from build123d import *

# Parameters (mm, degrees)
SKETCH2_R           = 50.8
SKETCH2_R_2         = 49.53
BOSS_EXTRUDE1_DEPTH = 304.8
CUT_EXTRUDE1_REACH  = 67.111
SKETCH3_W           = 80
SKETCH3_H           = 200
SKETCH7_R           = 1.5
CUT_EXTRUDE2_DEPTH  = 10


with BuildPart() as part:
    # Sketch2 → Boss-Extrude1 (new body)
    with BuildSketch(Plane.XY):
        Circle(SKETCH2_R)
        Circle(SKETCH2_R_2, mode=Mode.SUBTRACT)
    extrude(amount=BOSS_EXTRUDE1_DEPTH)

    # Sketch3 → Cut-Extrude1 (cut, up to next)
    with BuildSketch(Plane(origin=(0, 0, 0), x_dir=(0.939692621, -0.342020143, 0), z_dir=(0.342020143, 0.939692621, 0)), mode=Mode.PRIVATE) as cut_extrude1_sk1:
        with Locations((0, -152.4)):
            Rectangle(SKETCH3_W, SKETCH3_H)
    cut_extrude1_tool1 = extrude(cut_extrude1_sk1.sketch, amount=CUT_EXTRUDE1_REACH, mode=Mode.PRIVATE) & part.part
    add(cut_extrude1_tool1.solids().sort_by_distance((0, 0, 152.4))[0], mode=Mode.SUBTRACT)

    # Sketch7 → Cut-Extrude2 (cut)
    with BuildSketch(Plane(origin=(-78.038389788, 6.264218534, 0), x_dir=(-0.785593968, -0.618742367, 0), z_dir=(0.618742367, -0.785593968, 0))):
        with Locations((-57.430550893, -222.4)):
            Circle(SKETCH7_R)
        with Locations((-57.430550893, -197)):
            Circle(SKETCH7_R)
        with Locations((-57.430550893, -107.8)):
            Circle(SKETCH7_R)
        with Locations((-57.430550893, -82.4)):
            Circle(SKETCH7_R)
    extrude(amount=CUT_EXTRUDE2_DEPTH, mode=Mode.SUBTRACT)


solid = part.part
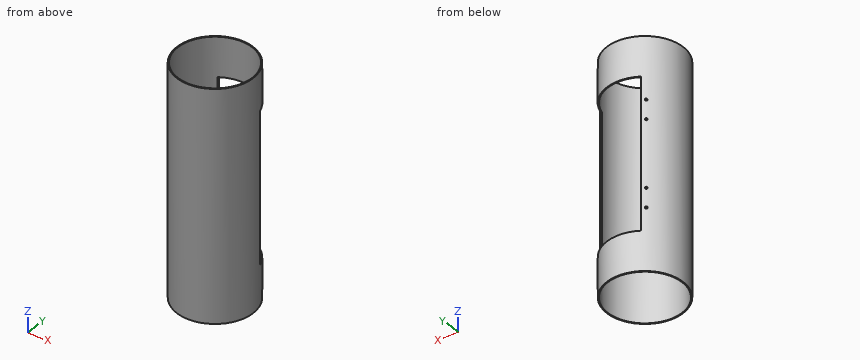
Geometry check sheet. Reference: the model listing, model coordinates, mm. Round coordinates to 2 decimals unless told otherwise and drop trailing zeros. Loops run counter-clockwise (first coordinate to the right, second up) from the corner with the lowest first, then second, coordinate; pieces in that order, holes last.
Item 1: Thickness scan on line 1 (X direction, y = 5, z = 189.5); line 2 (Y direction, x = 0, z = 144); line 3 (X direction, y = -39.5, z = 129). Record the ranges inside material, lowest first.
Item 2: Cross-section at C-C on z = 68.5. Record the boundary of the cut face in (x, y), then the cut area to 3 significant figures.
Item 3: Cross-section at D-D on x = -19.5. Record the boundary of the cut face in (y, z).
Item 4: Cross-section at A-A on x = 0. Record the boundary of the cut face in (y, z), then the cut area to 3 significant figures.
Item 5: Gauge pin test, flat ends, axial feed: pin 1 (3 mm diameter, centred on x = -15, z = 151, fed in from +Y); pin 2 (3 mm diameter, centred on y = -28, z = 81, fed in from -X); pin 3 (6 mm diameter, centred on x = 4, z = 132.5, fed in from +Y). Record the tip position at first contact, or that the pin passes through.
Item 6: Cross-section at B-B on y = 0. Record the boundary of the cut face in (x, z).
Answer sheet:
1. line 1: x = -50.55 to -49.28, 49.28 to 50.55
1. line 2: y = -50.8 to -49.53
1. line 3: x = -31.94 to -29.88, 29.88 to 31.94
2. outline: (-27.6, 41.13) - (-26.88, 43.11) arc R50.8 ccw (long way) to (48.3, 15.75) - (47.58, 13.77) arc R49.53 cw (long way) to start
2. area: 283 mm2
3. outline: (-46.91, 0) - (-45.53, 0) - (-45.53, 304.8) - (-46.91, 304.8) - close; (45.53, 0) - (46.91, 0) - (46.91, 52.4) - (45.53, 52.4) - close; (45.53, 252.4) - (46.91, 252.4) - (46.91, 304.8) - (45.53, 304.8) - close
4. outline: (-50.8, 0) - (-49.53, 0) - (-49.53, 304.8) - (-50.8, 304.8) - close; (49.53, 0) - (50.8, 0) - (50.8, 52.4) - (49.53, 52.4) - close; (49.53, 252.4) - (50.8, 252.4) - (50.8, 304.8) - (49.53, 304.8) - close
4. area: 520 mm2
5. pin 1: stops at y = -46.7
5. pin 2: stops at x = -43.34
5. pin 3: stops at y = -49.03
6. outline: (-50.8, 0) - (-49.53, 0) - (-49.53, 304.8) - (-50.8, 304.8) - close; (49.53, 0) - (50.8, 0) - (50.8, 304.8) - (49.53, 304.8) - close
